from build123d import *

# Parameters (mm, degrees)
BASE_FLANGE1_DEPTH           = 31.75
SKETCH6_R                    = 25.4
CUT_EXTRUDE1_DEPTH           = 166.905219101
FILLET1_R                    = 2.54
CUT_EXTRUDE2_DEPTH           = 90.31631094
F_7_0_201_DIAMETER_HOLE1_D   = 5.1054
F_25_0_1495_DIAMETER_HOLE1_D = 3.7973


# Sheet-metal steps are written as plain solids
with BuildPart() as part:
    # Sketch1 → Base-Flange1 (new, symmetric)
    with BuildSketch(Plane(origin=(0, 0, 0), x_dir=(-1, 0, 0), z_dir=(0, 1, 0))):
        with BuildLine():
            Line((9.525, -81.28), (9.525, 76.708))
            ThreePointArc((9.525, 76.708), (8.185892204, 79.940892204), (4.953, 81.28))
            Line((4.953, 81.28), (-9.525, 81.28))
            Line((-9.525, 81.28), (-9.525, 78.994))
            Line((-9.525, 78.994), (4.953, 78.994))
            ThreePointArc((4.953, 78.994), (6.569446102, 78.324446102), (7.239, 76.708))
            Line((7.239, 76.708), (7.239, -81.28))
            Line((7.239, -81.28), (9.525, -81.28))
        make_face()
    extrude(amount=BASE_FLANGE1_DEPTH, both=True)

    # Sketch6 → Cut-Extrude1 (cut, through all)
    with BuildSketch(Plane.XY.offset(81.28)):
        with Locations((22.225, 0)):
            Circle(SKETCH6_R)
    extrude(amount=-CUT_EXTRUDE1_DEPTH, mode=Mode.SUBTRACT)

    # Fillet1
    fillet1_edges = [part.edges().sort_by_distance(p)[0] for p in [
        (9.525, 31.75, 80.137),
        (9.525, -31.75, 80.137),
    ]]
    fillet(fillet1_edges, radius=FILLET1_R)

    # Sketch7 → Cut-Extrude2 (cut, through all)
    with BuildSketch(Plane(origin=(-9.525, 0, 0), x_dir=(0, -1, 0), z_dir=(-1, 0, 0))):
        with BuildLine():
            Line((-31.75, -49.53), (-31.75, -100.33))
            Line((-31.75, -100.33), (31.75, -100.33))
            Line((31.75, -100.33), (31.75, -49.53))
            ThreePointArc((31.75, -49.53), (0, -81.28), (-31.75, -49.53))
        make_face()
    extrude(amount=-CUT_EXTRUDE2_DEPTH, mode=Mode.SUBTRACT)

    # #7 (0.201) Diameter Hole1 (through all)
    with Locations(Plane.ZY.offset(9.525)):
        with Locations((-49.53, 0)):
            Hole(F_7_0_201_DIAMETER_HOLE1_D / 2)

    # #25 (0.1495) Diameter Hole1 (through all)
    with Locations(Plane.XY.offset(81.28)):
        with Locations((3.175, 25.4), (3.175, -25.4)):
            Hole(F_25_0_1495_DIAMETER_HOLE1_D / 2)


solid = part.part
The model under review builds one solid part; all positions refer to its coordinate system, in mm. A direction names the side the tool comes from. Coordinates: 2 decimals unless noted, no trailing zeros. Write each loop counter-clockwise with the first axis right and the second up, starting at its lowest first coordinate (ties: lowest second). Pieces come first, ordered by that corner, then holes. Notation, with made-up numbers: M 46.25,84.5 L 65.25,84.5 A15 cw 65.25,100.5 Z; hole C 85.5,69.5 d1. An arc over 180 degrees is marked long. Put each result on its own line as item: value.
1) Add section D-D on z = 46.5. Give the boundary of the cut face in (x, y) (3 decimals).
Computed:
outline: M -9.525,-31.75 L -7.239,-31.75 L -7.239,31.75 L -9.525,31.75 Z
2) Add section C-C on y = -25.4. Give the boundary of the cut face in (x, z) (3 decimals).
Computed:
outline: M -9.525,-68.58 L -7.239,-68.58 L -7.239,76.708 A2.286 cw -4.953,78.994 L 1.276,78.994 L 1.276,81.28 L -4.953,81.28 A4.572 ccw -9.525,76.708 Z; M 5.074,78.994 L 9.525,78.994 L 9.525,81.28 L 5.074,81.28 Z
3) Wall thickness on probe 1 along Y at (x, z) = (-8.05, -49.53); probe 2 along X at (y, z) = (12.5, 25) (3 decimals); probe 3 along Z at (x, y) = (7.5, 27.5): over which ranges is each line inside the solid? List them lowest first. Write a range as [from, to].
Computed:
probe 1: y = [-31.75, -2.55], [2.55, 31.75]
probe 2: x = [-9.525, -7.239]
probe 3: z = [78.99, 81.28]
4) Add section A-A on y = 0. Give the boundary of the cut face in (x, z) (3 decimals).
Computed:
outline: M -9.525,-81.28 L -7.239,-81.28 L -7.239,-52.083 L -9.525,-52.083 Z; M -9.525,-46.977 L -7.239,-46.977 L -7.239,76.708 A2.286 cw -4.953,78.994 L -3.175,78.994 L -3.175,81.28 L -4.953,81.28 A4.572 ccw -9.525,76.708 Z
5) For faces 1 (the cylindrical face through (2.15, 27, 80.12)), 2 (the flat face through (-4, 0, 78.994)), list the 3-axis set-ups (+Z, -Z, +X, -X, +Y, -Y) from which the entire face can be reached by the end or side of a thin tool; tool diameter is ignored.
Computed:
face 1: +Z, -Z
face 2: -Z, +X, +Y, -Y
6) Draft analysis for pull direction Y (two halves, no side actions). For faces 3 (the flat face through (-7.239, 0, -1)), 4 (the flat face through (-8, 31.75, 26)), 5 (the cylindrical face through (3.422, -23.518, 80.121)), state which applies: released by +Y, released by -Y, zero draft, split by the parting line, or undercut.
Computed:
face 3: zero draft
face 4: released by +Y
face 5: undercut
7) Clearance check with flat-ended pins moving along their axes: pin 1 Ø12 at (y, z) = (12, 3.5) entering from +X; pin 2 Ø4.5 at (x, y) = (3, -13.5) entering from -Z; pin 3 Ø3 at (x, y) = (3.175, -25.4) entering from +Z. State where each tip first meets the part, or that it passes through.
Computed:
pin 1: stops at x = -7.24
pin 2: stops at z = 78.99
pin 3: passes through
8) Add section B-B on x = 3. Give the boundary of the cut face in (y, z), then the cut area to 3 significant figures.
Computed:
outline: M -31.75,78.99 L -27.29,78.99 L -27.29,81.28 L -31.75,81.28 Z; M -23.51,78.99 L -16.6,78.99 L -16.6,81.28 L -23.51,81.28 Z; M 16.6,78.99 L 23.51,78.99 L 23.51,81.28 L 16.6,81.28 Z; M 27.29,78.99 L 31.75,78.99 L 31.75,81.28 L 27.29,81.28 Z
area: 52.0 mm2
